Geometry check sheet. Reference: the model listing, model coordinates, mm. A direction names the side the tool comes from. Round coordinates to 2 decimals unless told otherwise and drop trailing zeros. Order: outer loops, then holes, each group sorted by start corner. A loop starts at its lowest first (then second) coordinate and runs counter-clockwise, first axis right, second up.
```python
from build123d import *

# Parameters (mm, degrees)
F2_W     = 250
F2_H     = 232.13203
F3_DEPTH = 10
F5_DEPTH = 125
F6_W     = 20
F6_H     = 42.426406
F7_DEPTH = 20


# Not quite as in the source:
# - a pattern or mirror of a feature is missing from the dataset's text; its kind, count and spacing are read off the source's solid


with BuildPart() as f3:
    # F2 (on Right) → F3 (new body, symmetric)
    with BuildSketch(Plane.YZ):
        Rectangle(F2_W, F2_H)
    extrude(amount=F3_DEPTH, both=True)

    # F4 (on Front) → F5 (cut, symmetric)
    with BuildSketch(Plane.XZ):
        Polygon((10, 116.066015), (-10, 116.066015), (10, 96.066015), align=None)
        Polygon((-10, -116.066015), (10, -116.066015), (-10, -96.066015), align=None)
    extrude(amount=F5_DEPTH, both=True, mode=Mode.SUBTRACT)

    # F6 (on face) → F7 (cut)
    with BuildSketch(Plane.XZ.offset(125)):
        Polygon((-10, 53.639609), (10, 53.639609), (10, 96.066015), (-10, 116.066015), (-10, 96.066015), align=None)
        with Locations((0, -10)):
            Rectangle(F6_W, F6_H)
        with Locations((0, -94.852812)):
            Rectangle(F6_W, F6_H)
    f7 = extrude(amount=-F7_DEPTH, mode=Mode.SUBTRACT)

    # F7_copies: F7 across plane
    add(f7.mirror(Plane.ZX), mode=Mode.SUBTRACT)


solid = f3.part
```
(1) Material ranges on line 1 (Z direction, x = -2.75, y = 112.5); line 2 (Y direction, x = -5.5, z = -15); line 3 (Z direction, x = -2.5, y = -39), recorded low to high.
Returned:
line 1: z = -73.64 to -31.21, 11.21 to 53.64
line 2: y = -105 to 105
line 3: z = -103.57 to 108.57
(2) Draft check along Z on faces 4 (the flat face through (0, -115, -31.213)), 5 (the flat face through (0, 105, -10)), 6 (the flat face through (0, 105, -90)), 7 (the flat face through (0, -115, 53.64)). Enter one of: released by +Z, released by -Z, zero draft, split by the parting line, or undercut.
Returned:
face 4: undercut
face 5: undercut
face 6: zero draft
face 7: released by +Z
(3) Sectioned sample at B-B, the plane x = -5.5. Record the cut outline in (y, z), and give its area (3 significant figures).
Returned:
outline: (-125, -73.64) - (-105, -73.64) - (-105, -100.57) - (105, -100.57) - (105, -73.64) - (125, -73.64) - (125, -31.21) - (105, -31.21) - (105, 11.21) - (125, 11.21) - (125, 53.64) - (105, 53.64) - (105, 111.57) - (-105, 111.57) - (-105, 53.64) - (-125, 53.64) - (-125, 11.21) - (-105, 11.21) - (-105, -31.21) - (-125, -31.21) - close
area: 47,900 mm2
(4) Depth check by flat-ended pin: P1, Ø10, axis at x = -2, y = 119.5, coming from the +Z side; P2, Ø6, axis at x = -4, y = 118, coming from the -Z side; P3, Ø4, axis at x = -1, y = -69, coming from the -Z side. Enter the tip coordinate at first touch or a pass-through.
Returned:
P1: stops at z = 53.64
P2: stops at z = -73.64
P3: stops at z = -107.07
(5) Sectioned sample at A-A, the plane z = -19. Record the cut outline in (x, y), and give its area (3 significant figures).
Returned:
outline: (-10, -105) - (10, -105) - (10, 105) - (-10, 105) - close
area: 4,200 mm2
(6) Sectioned sample at C-C, the plane y = 97.5. Record the cut outline in (x, z), and give its area (3 significant figures).
Returned:
outline: (-10, -96.07) - (10, -116.07) - (10, 96.07) - (-10, 116.07) - close
area: 4,240 mm2
(7) Set-up check for faces 1 (the flat face through (0, -115, -73.64)), 2 (the flat face through (0, 105, 78)), 3 (the flat face through (0, -105, 78)): record each of +Z, -Z, +X, -X, +Y, -Y from which the full face is reachable in a straight line by a thin tool's end or side.
Returned:
face 1: -Z, +X, -X, -Y
face 2: +Z, +X, -X, +Y
face 3: +Z, +X, -X, -Y
